For this review, use the dimensioned drawing (mm, ordinates from the lowest corner) and the shaded views. Give positions to 0.01 mm unless a question says otherwise; leave off trailing zeros. Order: outer loops, then holes, each group sorted by start corner. A loop starts at its lowest first (then second) coordinate and runs counter-clockwise, first axis right, second up. Notation, with made-up numbers: (7.5, -12.5) - (18.5, -12.5) arc R4 ccw to (18.5, -5.5) - close; hole circle Ø6 at (40.5, -1). An arc over 180 degrees is marked (long way). Use a Markdown table: item, result. Add a question column.
1) We need section C-C on z = 6.5. Write out the cut boundary in (x, y) (1 decimal), then the cut area to 3 significant figures.
2) We need section A-A on y = 19.5. Write out the cut boundary in (x, z), then the cut area to 3 significant figures.
3) We need section B-B on x = 30. Write out the cut boundary in (y, z).
4) Wall thickness on L1, parallel to X at y = 21.5, z = 23.75; L2, parallel to X at y = 15.5, z = 3.5 (1 decimal); L3, parallel to Y at x = 30.5, z = 4.75: over which ranges is each line inside the solid? List them lowest first.
5) Clearance check with a flat-ended pin moving along its axis: P1, Ø12, axis at x = 28, y = 32.5, coming from the -Z side. State where the tip first meets the part, or that it passes through.
6) Mouldability with a two-part tool opening along X and no side actions: class the marked faces 1, 2 and 3 as released by +X, released by -X, zero draft, split by the parting line, or undercut.
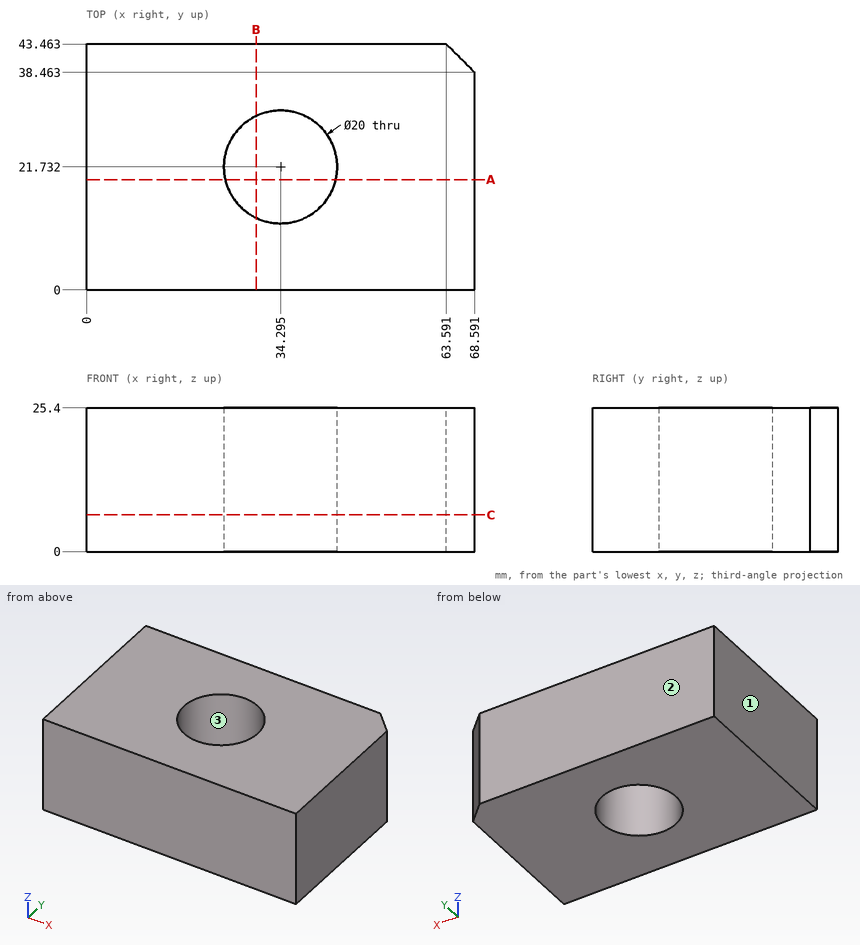
Checked values:
| question | item | result |
|---|---|---|
| 1 | outline | (0, 0) - (68.6, 0) - (68.6, 38.5) - (63.6, 43.5) - (0, 43.5) - close; hole circle Ø20 at (34.3, 21.7) |
| 1 | area | 2,650 mm² |
| 2 | outline | (0, 0) - (24.55, 0) - (24.55, 25.4) - (0, 25.4) - close; (44.04, 0) - (68.59, 0) - (68.59, 25.4) - (44.04, 25.4) - close |
| 2 | area | 1,250 mm² |
| 3 | outline | (0, 0) - (12.7, 0) - (12.7, 25.4) - (0, 25.4) - close; (30.76, 0) - (43.46, 0) - (43.46, 25.4) - (30.76, 25.4) - close |
| 4 | L1 | 0 to 24.3, 44.29 to 68.59 |
| 4 | L2 | 0 to 26.5, 42.1 to 68.6 |
| 4 | L3 | 0 to 12.48, 30.98 to 43.46 |
| 5 | P1 | z = 0 |
| 6 | face 1 | released by -X |
| 6 | face 2 | zero draft |
| 6 | face 3 | undercut |
